```python
from build123d import *

# Parameters (mm, degrees)
SKETCH1_W                                     = 208
SKETCH1_H                                     = 208
BASE_PLATE_DEPTH                              = 4
MOUNTING_HOLES_START                          = 1.5
MOUNTING_HOLES_OUTLINE_R                      = 3.25
MOUNTING_HOLES_DEPTH                          = 2.5
MOUNTING_HOLES_2_OUTLINE_R                    = 1.7
MOUNTING_HOLES_2_DEPTH                        = 1.5
MOUNTING_HOLES_MIRROR2_START                  = 1.5
MOUNTING_HOLES_MIRROR2_COPY_1_SKETCH_R        = 3.25
MOUNTING_HOLES_MIRROR2_COPY_1_DEPTH           = 2.5
MOUNTING_HOLES_MIRROR2_COPY_2_SKETCH_R        = 1.7
MOUNTING_HOLES_MIRROR2_COPY_2_DEPTH           = 1.5
MOUNTING_HOLES_MIRROR2_COPY_3_SKETCH_R        = 1.7
MOUNTING_HOLES_MIRROR2_COPY_3_DEPTH           = 1.5
SKETCH5_W                                     = 128
SKETCH5_H                                     = 4
SIDE_EXTRUSION_DEPTH                          = 14
SIDE_EXTRUSION_FILLET_R                       = 1
SIDE_EXTRUSION_CHAMFER_SIZE                   = 2
SIDE_EXTRUSION_FILLET_OF_SIDE_EXTRUSION_R     = 1
SIDE_EXTRUSION_CHAMFER_OF_SIDE_EXTRUSION_SIZE = 2
SIDE_EXTRUSION_MIRROR2_START                  = -64
SIDE_EXTRUSION_MIRROR2_DEPTH                  = 128
SIDE_EXTRUSION_MIRROR2_2_DEPTH                = 128
EDGE_FILLETS_R                                = 3


# Read off the part's stored shape, not the designer's step: mounting_holes, side_extrusion_mirror2
with BuildPart() as part:
    # Sketch1 → base_plate (new body)
    with BuildSketch(Plane(origin=(0, 0, 0), x_dir=(1, 0, 0), z_dir=(0, 1, 0))):
        Rectangle(SKETCH1_W, SKETCH1_H)
    extrude(amount=BASE_PLATE_DEPTH)

    # mounting_holes outline → mounting_holes (cut)
    with BuildSketch(Plane(origin=(0, 0, 0), x_dir=(1, 0, 0), z_dir=(0, 1, 0)).offset(MOUNTING_HOLES_START)):
        with Locations((95, 80)):
            Circle(MOUNTING_HOLES_OUTLINE_R)
        with Locations((80, 95)):
            Circle(MOUNTING_HOLES_OUTLINE_R)
    mounting_holes = extrude(amount=MOUNTING_HOLES_DEPTH, mode=Mode.SUBTRACT)

    # mounting_holes 2 outline → mounting_holes 2 (cut)
    with BuildSketch(Plane(origin=(0, 0, 0), x_dir=(1, 0, 0), z_dir=(0, 1, 0))):
        with Locations((95, 80)):
            Circle(MOUNTING_HOLES_2_OUTLINE_R)
        with Locations((80, 95)):
            Circle(MOUNTING_HOLES_2_OUTLINE_R)
    mounting_holes_2 = extrude(amount=MOUNTING_HOLES_2_DEPTH, mode=Mode.SUBTRACT)

    # mounting_holes_mirror1: mounting_holes, mounting_holes 2 across plane
    add(mounting_holes.mirror(Plane.XY), mode=Mode.SUBTRACT)
    add(mounting_holes_2.mirror(Plane.XY), mode=Mode.SUBTRACT)

    # mounting_holes_mirror2: mounting_holes, mounting_holes 2 across plane
    add(mounting_holes.mirror(Plane(origin=(0, 0, 0), x_dir=(0, 0, 1), z_dir=(1, 0, 0))), mode=Mode.SUBTRACT)
    add(mounting_holes_2.mirror(Plane(origin=(0, 0, 0), x_dir=(0, 0, 1), z_dir=(1, 0, 0))), mode=Mode.SUBTRACT)

    # mounting_holes_mirror2 copy 1 sketch → mounting_holes_mirror2 copy 1 (cut)
    with BuildSketch(Plane(origin=(0, 0, 0), x_dir=(-1, 0, 0), z_dir=(0, 1, 0)).offset(MOUNTING_HOLES_MIRROR2_START)):
        with Locations((95, 80)):
            Circle(MOUNTING_HOLES_MIRROR2_COPY_1_SKETCH_R)
        with Locations((80, 95)):
            Circle(MOUNTING_HOLES_MIRROR2_COPY_1_SKETCH_R)
    extrude(amount=MOUNTING_HOLES_MIRROR2_COPY_1_DEPTH, mode=Mode.SUBTRACT)

    # mounting_holes_mirror2 copy 2 sketch → mounting_holes_mirror2 copy 2 (cut)
    with BuildSketch(Plane(origin=(0, 0, 0), x_dir=(-1, 0, 0), z_dir=(0, 1, 0))):
        with Locations((95, 80)):
            Circle(MOUNTING_HOLES_MIRROR2_COPY_2_SKETCH_R)
        with Locations((80, 95)):
            Circle(MOUNTING_HOLES_MIRROR2_COPY_2_SKETCH_R)
    extrude(amount=MOUNTING_HOLES_MIRROR2_COPY_2_DEPTH, mode=Mode.SUBTRACT)

    # mounting_holes_mirror2 copy 3 sketch → mounting_holes_mirror2 copy 3 (cut)
    with BuildSketch(Plane(origin=(0, 0, 0), x_dir=(-1, 0, 0), z_dir=(0, 1, 0))):
        with Locations((95, -80)):
            Circle(MOUNTING_HOLES_MIRROR2_COPY_3_SKETCH_R)
        with Locations((80, -95)):
            Circle(MOUNTING_HOLES_MIRROR2_COPY_3_SKETCH_R)
    extrude(amount=MOUNTING_HOLES_MIRROR2_COPY_3_DEPTH, mode=Mode.SUBTRACT)

    # Sketch5 → side_extrusion (add)
    with BuildSketch(Plane(origin=(0, 4, 0), x_dir=(1, 0, 0), z_dir=(0, 1, 0))):
        with Locations((0, 106)):
            Rectangle(SKETCH5_W, SKETCH5_H)
    side_extrusion = extrude(amount=-SIDE_EXTRUSION_DEPTH)

    # side_extrusion_fillet
    side_extrusion_fillet_edges = [part.edges().sort_by_distance(p)[0] for p in [
        (0, 4, -108),
    ]]
    fillet(side_extrusion_fillet_edges, radius=SIDE_EXTRUSION_FILLET_R)

    # side_extrusion_chamfer
    side_extrusion_chamfer_edges = [part.edges().sort_by_distance(p)[0] for p in [
        (0, -10, -108),
    ]]
    chamfer(side_extrusion_chamfer_edges, length=SIDE_EXTRUSION_CHAMFER_SIZE)

    # side_extrusion_mirror1: side_extrusion across plane
    add(side_extrusion.mirror(Plane(origin=(0, 0, 0), x_dir=(0.7071067811865476, 0, 0.7071067811865476), z_dir=(0.7071067811865477, 0, -0.7071067811865475))))

    # side_extrusion_fillet of side_extrusion
    side_extrusion_fillet_of_side_extrusion_edges = [part.edges().sort_by_distance(p)[0] for p in [
        (-108, 4, 0),
    ]]
    fillet(side_extrusion_fillet_of_side_extrusion_edges, radius=SIDE_EXTRUSION_FILLET_OF_SIDE_EXTRUSION_R)

    # side_extrusion_chamfer of side_extrusion
    side_extrusion_chamfer_of_side_extrusion_edges = [part.edges().sort_by_distance(p)[0] for p in [
        (-108, -10, 0),
    ]]
    chamfer(side_extrusion_chamfer_of_side_extrusion_edges, length=SIDE_EXTRUSION_CHAMFER_OF_SIDE_EXTRUSION_SIZE)

    # side_extrusion_mirror2 outline → side_extrusion_mirror2 (add)
    with BuildSketch(Plane.YZ.offset(SIDE_EXTRUSION_MIRROR2_START)):
        with BuildLine():
            Line((-8, 108), (-10, 106))
            Line((-10, 106), (-10, 104))
            Line((-10, 104), (4, 104))
            Line((4, 104), (4, 107))
            ThreePointArc((4, 107), (3.707106781, 107.707106781), (3, 108))
            Line((3, 108), (-8, 108))
        make_face()
    extrude(amount=SIDE_EXTRUSION_MIRROR2_DEPTH)

    # side_extrusion_mirror2 2 outline → side_extrusion_mirror2 2 (add)
    with BuildSketch(Plane.XY.offset(SIDE_EXTRUSION_MIRROR2_START)):
        with BuildLine():
            Line((104, 4), (104, -10))
            Line((104, -10), (106, -10))
            Line((106, -10), (108, -8))
            Line((108, -8), (108, 3))
            ThreePointArc((108, 3), (107.707106781, 3.707106781), (107, 4))
            Line((107, 4), (104, 4))
        make_face()
    extrude(amount=SIDE_EXTRUSION_MIRROR2_2_DEPTH)

    # edge_fillets
    edge_fillets_edges = [part.edges().sort_by_distance(p)[0] for p in [
        (104, 2, 104),
        (-104, 2, 104),
        (-104, 2, -104),
        (104, 2, -104),
    ]]
    fillet(edge_fillets_edges, radius=EDGE_FILLETS_R)


solid = part.part
```
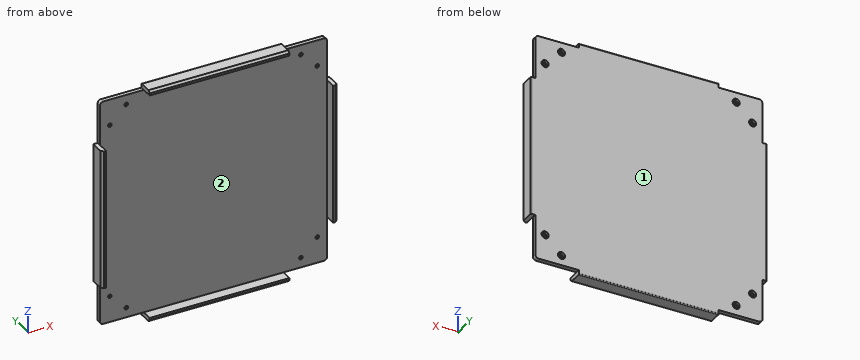
The listing builds one solid part. Answer for the finished solid, in the listing's coordinates (mm). Face numbers are marked on the shaded views. Give positions to 0.01 mm unless a question says otherwise; leave off trailing zeros. Order: outer loops, then holes, each group sorted by start corner. A loop starts at its lowest first (then second) coordinate and runs counter-clockwise, first axis right, second up. Notation, with made-up numbers: (54, 38.25) - (81, 38.25) arc R18 cw to (81, 71.25) - close; hole circle Ø11 at (-7, 9.5). An arc over 180 degrees is marked (long way). Answer in a Markdown table with one row per item. Add a question column.
Q1. Find the intervals of material crossed by line 1 along X through (y, z) = (2.65, -95); line 2 along X through (y, z) = (2, -80); line 3 along Z through (x, y) = (-80, 0.65), in increasing order. Write a range as [from, to].
Q2. The part is cut by section A-A (y = -4.5). Determine the outline of the cut face in (x, z).
Q3. The part is cut by section D-D (z = 68). Determine the outline of the cut face in (x, y), then the cut area to 3 significant figures.
Q4. For a pull along Z with two mould halves and no side action, classify the marked faces 1 and 2 as released by +Z, released by -Z, zero draft, split by the parting line, or undercut.
Q5. Given P1, Ø1.2, axis at x = -79.5, y = 1.5, coming from the -Z side; P2, Ø1.2, axis at y = 2, z = 75, coming from the -X side; P3, Ø1.5, axis at x = -28.5, z = 32, coming from the -Y side, each flat-ended and moving along its own axis, determine where each tip first touches the part or whether it passes through.
Q6. The part is cut by section B-B (x = -32). Determine the outline of the cut face in (y, z).
Q7. The part is cut by section C-C (z = -25.5). Determine the outline of the cut face in (x, y).
Determined:
| question | item | result |
|---|---|---|
| 1 | line 1 | x = [-104, -83.25], [-76.75, 76.75], [83.25, 104] |
| 1 | line 2 | x = [-104, -98.25], [-91.75, 91.75], [98.25, 104] |
| 1 | line 3 | z = [-104, -96.7], [-93.3, 93.3], [96.7, 104] |
| 2 | outline | (-108, -64) - (-104, -64) - (-104, 64) - (-108, 64) - close; (-64, -108) - (64, -108) - (64, -104) - (-64, -104) - close; (-64, 104) - (64, 104) - (64, 108) - (-64, 108) - close; (104, -64) - (108, -64) - (108, 64) - (104, 64) - close |
| 3 | outline | (-104, 0) - (104, 0) - (104, 4) - (-104, 4) - close |
| 3 | area | 832 mm² |
| 4 | face 1 | zero draft |
| 4 | face 2 | undercut |
| 5 | P1 | stops at z = -104 |
| 5 | P2 | stops at x = -104 |
| 5 | P3 | stops at y = 0 |
| 6 | outline | (-10, -106) - (-8, -108) - (3, -108) arc R1 ccw to (4, -107) - (4, 107) arc R1 ccw to (3, 108) - (-8, 108) - (-10, 106) - (-10, 104) - (0, 104) - (0, -104) - (-10, -104) - close |
| 7 | outline | (-108, -8) - (-106, -10) - (-104, -10) - (-104, 0) - (104, 0) - (104, -10) - (106, -10) - (108, -8) - (108, 3) arc R1 ccw to (107, 4) - (-107, 4) arc R1 ccw to (-108, 3) - close |
